Source: CAD feature listing. Evaluate the final solid. Frame: model axes, mm. Face numbers are marked on the shaded views. A direction names the side the tool comes from. Give positions to 0.01 mm unless a question says otherwise; leave off trailing zeros. Write each loop counter-clockwise with the first axis right and the second up, starting at its lowest first coordinate (ties: lowest second). Pieces come first, ordered by that corner, then holes. Notation, with made-up numbers: (-40, 66.25) -> (13, 66.25) arc R31 cw to (13, 96.25) -> close; hole circle Ø1 at (47, -14.75). An arc over 180 degrees is marked (long way). Answer as a JSON object with one key per item and string values. Group by question number.
Item 1: Pull-direction query (Z, two-part tool) for the marked faces 4, 5 and 6; classes: pulls with the +Z half, pulls with the -Z half, needs draft (parallel to the pull), parting line crosses it, or undercut.
Item 2: Section query A-A on z = -6. Return the cut outline in (x, y), plus the area to 3 significant figures.
Item 3: Section query C-C on y = 11.5. Return the cut outline in (x, z), plus the area to 3 significant figures.
Item 4: Ray query, probe 1 along Y at (x, z) = (-3.5, -0.5); probe 2 along Y at (x, z) = (-3.75, -13); probe 3 along X at (y, z) = (-21.2, -10). Return the intervals inside material, ascending. Write a range as from..to.
Item 5: Section query B-B on x = -7.5. Return the cut outline in (y, z), plus the area to 3 significant figures.
Item 6: Access query for the marked faces 1, 2 and 3. Directions: +Z, -Z, +X, -X, +Y, -Y. A direction counts if a zero-diameter tool reaches every point of the face in a straight line with its end or side. Return the directions, or none.
Item 7: First-contact query: pin 1 Ø12.5 at (x, y) = (-4, 2) entering from -Z; pin 2 Ø4 at (x, z) = (3, -18.5) entering from -Y; pin 3 Ø1 at (x, z) = (-9, 1) entering from +Y; pin 4 Ø2 at (x, z) = (-1, 19) entering from +Y. Flat tips, straight axial feed; report the tip coordinate or a pass-through.
Item 8: Section query D-D on z = 20.5. Return the cut outline in (x, y).
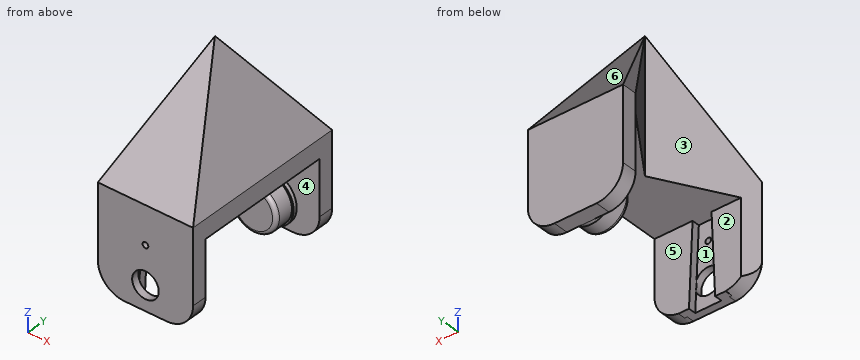
from build123d import *
from OCP.BRepFilletAPI import BRepFilletAPI_MakeChamfer

# Parameters (mm, degrees)
SKETCH4_W                = 12.46
SKETCH4_H                = 17.25
BOSS_EXTRUDE3_DEPTH      = 6
BOSS_EXTRUDE6_DEPTH      = 7.3
BOSS_EXTRUDE6_DEPTH_BACK = 17.25
SKETCH8_R                = 12.546781182
SKETCH8_R_2              = 11.15
BOSS_EXTRUDE4_DEPTH      = 17.25
SKETCH6_R                = 2
CUT_EXTRUDE1_DEPTH       = 5
CHAMFER1_SIZE            = 0.5
CHAMFER1_SIZE_2          = 0.866025404
SKETCH10_W               = 12.46
SKETCH10_H               = 23.7
CUT_EXTRUDE3_DEPTH       = 17.25
CUT_EXTRUDE4_REACH       = 43.938
SKETCH11_W               = 5
SKETCH11_H               = 3
BOSS_EXTRUDE7_START      = -7.3
BOSS_EXTRUDE7_DEPTH      = 7.3
BOSS_EXTRUDE9_START      = 10
BOSS_EXTRUDE9_DEPTH      = 10
BOSS_EXTRUDE10_DEPTH     = 25.093562364
SKETCH18_W               = 21.5
SKETCH18_H               = 12.438292938
CUT_EXTRUDE5_DEPTH       = 2
CUT_EXTRUDE6_DEPTH       = 58.154608998
CUT_EXTRUDE6_DEPTH_BACK  = 58.154608998
SKETCH19_R               = 3.5
FILLET1_R                = 7
CUT_EXTRUDE7_DEPTH       = 55.97840444
CUT_EXTRUDE7_DEPTH_BACK  = 55.97840444
SKETCH20_W               = 25.093562364
SKETCH20_H               = 36.096781182
BOSS_EXTRUDE11_DEPTH     = 44.5
CUT_EXTRUDE8_DEPTH       = 40.401576339
CUT_EXTRUDE8_DEPTH_BACK  = 40.401576339
CUT_EXTRUDE9_DEPTH       = 40.401576339
CUT_EXTRUDE9_DEPTH_BACK  = 40.401576339
SKETCH24_R               = 6.5
BOSS_EXTRUDE12_DEPTH     = 5
SKETCH25_R               = 6.075
BOSS_EXTRUDE13_DEPTH     = 5
FILLET2_R                = 1
BOSS_EXTRUDE14_DEPTH     = 2
CUT_EXTRUDE10_REACH      = 57.104
SKETCH27_R               = 0.75


with BuildPart() as part:
    # Sketch4 → Boss-Extrude3 (new body)
    with BuildSketch(Plane.XY):
        with Locations((0, -1.35)):
            Rectangle(SKETCH4_W, SKETCH4_H)
    extrude(amount=BOSS_EXTRUDE3_DEPTH)



with BuildPart() as body_2:
    # Sketch8 → Boss-Extrude6 (new, two sides: drawn at the far end of the back side and taken through both)
    with BuildSketch(Plane(origin=(0, -9.975, 0), x_dir=(-1, 0, 0), z_dir=(0, -1, 0)).offset(-BOSS_EXTRUDE6_DEPTH_BACK)):
        with Locations(Location((0, -23.55, 0), (0, 0, 90))):
            Circle(SKETCH8_R)
        with Locations(Location((0, -23.55, 0), (0, 0, 90))):
            Circle(SKETCH8_R_2, mode=Mode.SUBTRACT)
    extrude(amount=BOSS_EXTRUDE6_DEPTH + BOSS_EXTRUDE6_DEPTH_BACK)


with BuildPart() as part_1:
    add(part.part)

    add(body_2.part)  # Boss-Extrude4 merges body 2
    # Sketch5 → Boss-Extrude4 (add)
    with BuildSketch(Plane(origin=(0, 7.275, 0), x_dir=(1, 0, 0), z_dir=(0, 1, 0))):
        with BuildLine():
            Line((12.546781182, -23.55), (12.546781182, 0))
            Line((12.546781182, 0), (6.23, 0))
            Line((6.23, 0), (6.23, -29.7))
            Line((6.23, -29.7), (-6.23, -29.7))
            Line((-6.23, -29.7), (-6.23, 0))
            Line((-6.23, 0), (-12.546781182, 0))
            Line((-12.546781182, 0), (-12.546781182, -23.55))
            ThreePointArc((-12.546781182, -23.55), (0, -36.096781182), (12.546781182, -23.55))
        make_face()
    extrude(amount=-BOSS_EXTRUDE4_DEPTH)

    # Sketch6 → Cut-Extrude1 (cut)
    with BuildSketch(Plane(origin=(0, 7.275, 0), x_dir=(1, 0, 0), z_dir=(0, 1, 0))):
        with Locations(Location((0, -3.5, 0), (0, 0, 270))):
            Circle(SKETCH6_R)
        with Locations(Location((0, -32.2, 0), (0, 0, 270))):
            Circle(SKETCH6_R)
    extrude(amount=-CUT_EXTRUDE1_DEPTH, mode=Mode.SUBTRACT)

    # Chamfer1
    chamfer1_edges_1 = [part_1.edges().sort_by_distance(p)[0] for p in [
        (0, 7.275, 1.5),
    ]]
    chamfer1_side_1 = [part_1.faces().sort_by_distance(p)[0] for p in [
        (0, 7.275, 1.49),
    ]]
    chamfer1_edges_2 = [part_1.edges().sort_by_distance(p)[0] for p in [
        (0, 7.275, 30.2),
    ]]
    chamfer1_side_2 = [part_1.faces().sort_by_distance(p)[0] for p in [
        (0, 7.275, 30.19),
    ]]
    chamfer1 = BRepFilletAPI_MakeChamfer(part_1.part.solid().wrapped)
    for e in chamfer1_edges_1:
        chamfer1.Add(CHAMFER1_SIZE - 0.0001, CHAMFER1_SIZE_2 - 0.0001, e.wrapped, chamfer1_side_1[0].wrapped)
    for e in chamfer1_edges_2:
        chamfer1.Add(CHAMFER1_SIZE - 0.0001, CHAMFER1_SIZE_2 - 0.0001, e.wrapped, chamfer1_side_2[0].wrapped)
    add(Compound.cast(chamfer1.Shape()), mode=Mode.REPLACE)  # a hair under: the kernel refuses the full size

    # Sketch10 → Cut-Extrude3 (cut)
    with BuildSketch(Plane(origin=(0, 7.275, 0), x_dir=(1, 0, 0), z_dir=(0, 1, 0))):
        with Locations((0, -17.85)):
            Rectangle(SKETCH10_W, SKETCH10_H)
    extrude(amount=-CUT_EXTRUDE3_DEPTH, mode=Mode.SUBTRACT)

    # Sketch11 → Cut-Extrude4 (cut, up to next)
    with BuildSketch(Plane.XY.offset(36.096781182), mode=Mode.PRIVATE) as cut_extrude4_sk1:
        with Locations((0, -8.475)):
            Rectangle(SKETCH11_W, SKETCH11_H)
    cut_extrude4_tool1 = extrude(cut_extrude4_sk1.sketch, amount=-CUT_EXTRUDE4_REACH, mode=Mode.PRIVATE) & part_1.part
    add(cut_extrude4_tool1.solids().sort_by_distance((0, -8.475, 36.096781))[0], mode=Mode.SUBTRACT)

    # Sketch13 → Boss-Extrude7 (add)
    with BuildSketch(Plane.XZ.offset(17.275).offset(BOSS_EXTRUDE7_START)):
        with BuildLine():
            Line((-12.546781182, 23.55), (-12.546781182, 0))
            Line((-12.546781182, 0), (12.546781182, 0))
            Line((12.546781182, 0), (12.546781182, 23.55))
            ThreePointArc((12.546781182, 23.55), (0, 11.003218818), (-12.546781182, 23.55))
        make_face()
    extrude(amount=BOSS_EXTRUDE7_DEPTH)

    # Sketch15 → Boss-Extrude9 (add)
    with BuildSketch(Plane(origin=(0, 7.275, 0), x_dir=(1, 0, 0), z_dir=(0, 1, 0)).offset(BOSS_EXTRUDE9_START)):
        with BuildLine():
            Line((-12.546781182, 0), (12.546781182, 0))
            Line((12.546781182, 0), (12.546781182, -23.55))
            ThreePointArc((12.546781182, -23.55), (0, -36.096781182), (-12.546781182, -23.55))
            Line((-12.546781182, -23.55), (-12.546781182, 0))
        make_face()
        with BuildLine():
            Line((-6.23, -0.8), (6.23, -0.8))
            Line((6.23, -0.8), (6.23, -33.5))
            ThreePointArc((6.23, -33.5), (5.937106781, -34.207106781), (5.23, -34.5))
            Line((5.23, -34.5), (-5.23, -34.5))
            ThreePointArc((-5.23, -34.5), (-5.937106781, -34.207106781), (-6.23, -33.5))
            Line((-6.23, -33.5), (-6.23, -0.8))
        make_face(mode=Mode.SUBTRACT)
    extrude(amount=-BOSS_EXTRUDE9_DEPTH)

    # Sketch17 → Boss-Extrude10 (add)
    with BuildSketch(Plane(origin=(-12.546781182, 4.728218818, 0), x_dir=(0, -1, 0), z_dir=(1, 0, 0))):
        Polygon((26.978218818, 26.5), (26.978218818, 0), (-17.521781182, 0), (-17.521781182, 26.5), (-13.521781182, 26.5), (-13.521781182, 5), (22.978218818, 5), (22.978218818, 26.5), align=None)
    extrude(amount=BOSS_EXTRUDE10_DEPTH)

    # Sketch18 → Cut-Extrude5 (cut)
    with BuildSketch(Plane.ZX.offset(-18.25)):
        with Locations((-15.75, 0)):
            Rectangle(SKETCH18_W, SKETCH18_H)
    extrude(amount=-CUT_EXTRUDE5_DEPTH, mode=Mode.SUBTRACT)

    # Sketch19 → Cut-Extrude6 (cut, two sides: drawn at the far end of the back side and taken through both)
    with BuildSketch(Plane.ZX.offset(-20.25).offset(-CUT_EXTRUDE6_DEPTH_BACK)):
        with Locations((-20, 0)):
            Circle(SKETCH19_R)
    extrude(amount=CUT_EXTRUDE6_DEPTH + CUT_EXTRUDE6_DEPTH_BACK, mode=Mode.SUBTRACT)

    # Fillet1
    fillet1_edges = [part_1.edges().sort_by_distance(p)[0] for p in [
        (12.546781182, -20.25, -26.5),
        (-12.546781182, -20.25, -26.5),
        (-12.546781182, 20.25, -26.5),
        (12.546781182, 20.25, -26.5),
    ]]
    fillet(fillet1_edges, radius=FILLET1_R)

    # Sketch20 → Cut-Extrude7 (cut, two sides: drawn at the far end of the back side and taken through both)
    with BuildSketch(Plane(origin=(0, 17.275, 0), x_dir=(1, 0, 0), z_dir=(0, 1, 0)).offset(-CUT_EXTRUDE7_DEPTH_BACK)):
        with Locations((0, -18.048390591)):
            Rectangle(SKETCH20_W, SKETCH20_H)
    extrude(amount=CUT_EXTRUDE7_DEPTH + CUT_EXTRUDE7_DEPTH_BACK, mode=Mode.SUBTRACT)

    # Sketch21 → Boss-Extrude11 (add)
    with BuildSketch(Plane(origin=(0, 22.25, 0), x_dir=(1, 0, 0), z_dir=(0, 1, 0))):
        Polygon((12.546781182, 0), (-0.025415104, -30), (-12.546781182, 0), align=None)
    extrude(amount=-BOSS_EXTRUDE11_DEPTH)

    # Sketch22 → Cut-Extrude8 (cut, two sides: drawn at the far end of the back side and taken through both)
    with BuildSketch(Plane(origin=(0, 0, 0), x_dir=(0, 0, -1), z_dir=(1, 0, 0)).offset(-CUT_EXTRUDE8_DEPTH_BACK)):
        Polygon((0, 22.25), (-30, 0.01), (-30, 22.25), align=None)
        Polygon((0, -22.25), (-30, -22.25), (-30, -0.01), align=None)
    extrude(amount=CUT_EXTRUDE8_DEPTH + CUT_EXTRUDE8_DEPTH_BACK, mode=Mode.SUBTRACT)

    # Sketch23 → Cut-Extrude9 (cut, two sides: drawn at the far end of the back side and taken through both)
    with BuildSketch(Plane(origin=(0, 0, 0), x_dir=(-1, 0, 0), z_dir=(0, 0, -1)).offset(-CUT_EXTRUDE9_DEPTH_BACK)):
        Polygon((12.546781182, 18.25), (0, 0), (12.546781182, -22.25), align=None)
    extrude(amount=CUT_EXTRUDE9_DEPTH + CUT_EXTRUDE9_DEPTH_BACK, mode=Mode.SUBTRACT)

    # Sketch24 → Boss-Extrude12 (add)
    with BuildSketch(Plane(origin=(0, 22.25, 0), x_dir=(1, 0, 0), z_dir=(0, 1, 0))):
        with Locations(Location((0, 20, 0), (0, 0, 270))):
            Circle(SKETCH24_R)
    extrude(amount=-BOSS_EXTRUDE12_DEPTH)

    # Sketch25 → Boss-Extrude13 (add)
    with BuildSketch(Plane.XZ.offset(-17.25)):
        with Locations(Location((0, -20, 0), (0, 0, 270))):
            Circle(SKETCH25_R)
    extrude(amount=BOSS_EXTRUDE13_DEPTH)

    # Fillet2
    fillet2_edges = [part_1.edges().sort_by_distance(p)[0] for p in [
        (0, 12.25, -13.925),
    ]]
    fillet(fillet2_edges, radius=FILLET2_R)

    # Sketch26 → Boss-Extrude14 (add)
    with BuildSketch(Plane(origin=(0, -20.25, 0), x_dir=(1, 0, 0), z_dir=(0, 1, 0))):
        Polygon((-6.219146469, 5), (-2.5, 5), (-3.1585, 20), (-3.44385, 26.5), (-6.219146469, 26.5), align=None)
        Polygon((3.1585, 20), (3.44385, 26.5), (6.219146469, 26.5), (6.219146469, 5), (2.5, 5), align=None)
    extrude(amount=BOSS_EXTRUDE14_DEPTH)

    # Sketch27 → Cut-Extrude10 (cut, up to next)
    with BuildSketch(Plane.XZ.offset(22.25), mode=Mode.PRIVATE) as cut_extrude10_sk1:
        with Locations(Location((0, -10, 0), (0, 0, 270))):
            Circle(SKETCH27_R)
    cut_extrude10_tool1 = extrude(cut_extrude10_sk1.sketch, amount=-CUT_EXTRUDE10_REACH, mode=Mode.PRIVATE) & part_1.part
    add(cut_extrude10_tool1.solids().sort_by_distance((0, -22.25, -10))[0], mode=Mode.SUBTRACT)


solid = part_1.part
Worked answers:
{
 "1": {"face 4": "undercut", "face 5": "needs draft", "face 6": "pulls with the +Z half"},
 "2": {"outline": "(-12.55, -22.25) -> (12.55, -22.25) -> (12.55, -18.25) -> (2.54, -18.25) -> (2.54, -20.25) -> (-2.54, -20.25) -> (-2.54, -18.25) -> (-10.29, -18.25) -> close; (-12.55, 18.25) -> (12.55, 18.25) -> (12.55, 22.25) -> (-12.55, 22.25) -> close", "area": "186 mm^2"},
 "3": {"outline": "(-7.91, -5) -> (12.55, -5) -> (12.55, 0) -> (6.47, 14.5) -> (-6.49, 14.5) -> (-7.91, 11.12) -> close", "area": "352 mm^2"},
 "4": {"probe 1": "-22.25..-6.21, 5.09..22.25", "probe 2": "-22.25..-18.25, 18.25..22.25", "probe 3": "-11.95..-0.75, 0.75..12.55"},
 "5": {"outline": "(-22.25, -26.22) -> (-18.25, -26.22) -> (-18.25, -5) -> (-13.3, -5) -> (-13.3, 12.07) -> (-22.25, 0) -> close; (10.91, -5) -> (18.25, -5) -> (18.25, -26.22) -> (22.25, -26.22) -> (22.25, 0) -> (13.29, 12.09) -> (10.91, 12.09) -> close", "area": "408 mm^2"},
 "6": {"face 1": "-Z", "face 2": "-Z, +X, -X", "face 3": "+Z, -Z, -X"},
 "7": {"pin 1": "z = -5", "pin 2": "y = -22.25", "pin 3": "y = 21.88", "pin 4": "y = 8.91"},
 "8": {"outline": "(-3.99, 5.8) -> (0, 0) -> (-3.98, -7.05) -> (3.96, -7.05) -> (3.96, 7.05) -> (-3.99, 7.05) -> close"}
}
